from build123d import *

# Parameters (mm, degrees)
F1_DEPTH = 18
F2_R     = 7.5
F3_DEPTH = 19.001
F4_R     = 7.5
F5_DEPTH = 25
F6_R     = 0.99999


# Not quite as in the source:
# - a fillet or chamfer is up to 0.001 mm smaller than in the source, because OpenCascade refuses the exact size


with BuildPart() as f1:
    # F0 (on Top) → F1 (new body)
    with BuildSketch(Plane.XY):
        with BuildLine():
            ThreePointArc((11.5, 0), (0, -11.5), (-11.5, 0))
            Line((-11.5, 0), (-11.5, 5))
            Line((-11.5, 5), (-14, 5))
            Line((-14, 5), (-14, 0))
            ThreePointArc((-14, 0), (0, -14), (14, 0))
            Line((14, 0), (15, 0))
            Line((15, 0), (15, 12.5))
            Line((15, 12.5), (9.5, 12.5))
            Line((9.5, 12.5), (9.5, 10))
            Line((9.5, 10), (12.5, 10))
            Line((12.5, 10), (12.5, 4.5))
            Line((12.5, 4.5), (11.5, 4.5))
            Line((11.5, 4.5), (11.5, 0))
        make_face()
    extrude(amount=F1_DEPTH)

    # F2 (on face) → F3 (cut, through all)
    with BuildSketch(Plane(origin=(0, 5, 0), x_dir=(-1, 0, 0), z_dir=(0, 1, 0))):
        with Locations((20, 9)):
            Circle(F2_R)
    extrude(amount=-F3_DEPTH, mode=Mode.SUBTRACT)

    # F4 (on face) → F5 (cut)
    with BuildSketch(Plane.YZ.offset(-11.5)):
        with Locations((11, 9)):
            Circle(F4_R)
    extrude(amount=-F5_DEPTH, mode=Mode.SUBTRACT)

    # F6 (radius 1 in the source; OpenCascade refuses exactly that, so slightly less here)
    f6_edges = [f1.edges().sort_by_distance(p)[0] for p in [
        (-11.5, 5, 15.75),
        (-11.5, 5, 2.25),
        (12.5, 4.5, 9),
        (12.5, 10, 9),
        (9.5, 12.5, 9),
    ]]
    fillet(f6_edges, radius=F6_R)


solid = f1.part
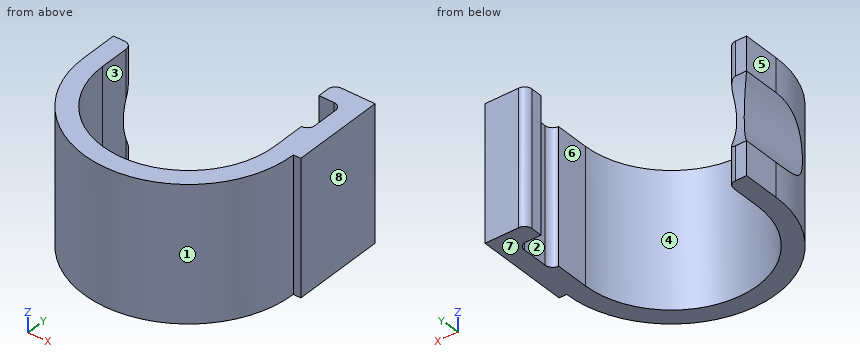
Model file for the job. Use its own axes, mm. Face numbers are marked on the shaded views. A direction names the side the tool comes from. Give positions to 0.01 mm unless a question says otherwise; leave off trailing zeros. Loops run counter-clockwise (first coordinate to the right, second up) from the corner with the lowest first, then second, coordinate; pieces in that order, holes last.
1) Pull direction X, two halves, no side cores. Call the marked faces 6, 7 and 8: +X half, -X half, draft (parallel to the pull), parting line (faces both ways), or undercut.
2) Tool access for the marked faces 1, 2, 3, 4 and 5: list every direction of +Z, -Z, +X, -X, +Y, -Y with a clear straight run to the whole face (end or side of a thin tool).
3) Saw through at A-A (y = -1.5). Write the cut outline in (x, z).
4) Saw through at C-C (y = -8.75). Write the cut outline in (x, z).
5) Saw through at D-D (x = 0). Write the cut outline in (y, z).
6) Wall check: line 1 (X direction, y = 2, z = 3.25); line 2 (X direction, y = 9, z = 16.75); line 3 (X direction, y = -9.25, z = 15.75). Give the ranges that are in metal, low to high.
7) Flat gauge pins, fed straight in: pin 1 Ø0.8 at (x, z) = (-13.5, 1.5) entering from +Y; pin 2 Ø0.6 at (x, z) = (10.5, 13) entering from -Y; pin 3 Ø6 at (y, z) = (-6, 3.5) entering from +X. Where does each tip first touch, or does it go through?
Answer block:
1. face 6: undercut
1. face 7: draft
1. face 8: +X half
2. face 1: +Z, -Z, -Y
2. face 2: +Z, -Z, -X
2. face 3: +Z, -Z, +Y
2. face 4: +Z, -Z
2. face 5: +Z, -Z, -X, +Y, -Y
3. outline: (-13.92, 0) - (-11.4, 0) - (-11.4, 18) - (-13.92, 18) - (-13.92, 13.39) arc R7.5 cw to (-13.92, 4.61) - close; (11.4, 0) - (13.92, 0) - (13.92, 18) - (11.4, 18) - close
4. outline: (-10.93, 0) - (-7.46, 0) - (-7.46, 18) - (-10.93, 18) - close; (7.46, 0) - (10.93, 0) - (10.93, 18) - (7.46, 18) - close
5. outline: (-14, 0) - (-11.5, 0) - (-11.5, 18) - (-14, 18) - close
6. line 1: x = -14 to -11.5, 11.5 to 15
6. line 2: x = 12.5 to 15
6. line 3: x = -10.51 to -6.83, 6.83 to 10.51
7. pin 1: stops at y = 5
7. pin 2: stops at y = -9.59
7. pin 3: stops at x = 13.67
